Autodesk Inventor part; units mm, degrees
ref_plane "YZ Plane" through (0, 0, 0) normal (1, 0, 0) x (0, 1, 0)
ref_plane "XZ Plane" through (0, 0, 0) normal (0, 1, 0) x (-1, 0, 0)
ref_plane "XY Plane" through (0, 0, 0) normal (0, 0, 1) x (1, 0, 0)
sketch "スケッチ1" plane through (0, 0, 0) normal (0, 0, 1) x (1, 0, 0)
  line L0 (-22, 0) -> (22, 0)
  line L1 (22, 0) -> (22, 17)
  line L2 (22, 17) -> (-22, 17)
  line L3 (-22, 17) -> (-22, 0)
  point P0 (0, 0)
  point P1 (0, 0)
  dimension "d0" = 44
  dimension "d1" = 17
extrude "土台" add sketch "スケッチ1" along normal blind 2
sketch "スケッチ2" plane through (-22, 0, 0) normal (0, -1, 0) x (1, 0, 0)
  line L0 (22, 0) -> (22, 53.3234) construction
  circle A0 centre (22, 25) radius 15 construction
  line L1 (0, 2) -> (44, 2) construction
  line L2 (-7.4711, 25) -> (51.4711, 25) construction
  circle A1 centre (3.5, 25) radius 1.6
  circle A2 centre (40.5, 25) radius 1.6
  line L3 (0, 2) -> (7, 2)
  line L4 (7, 2) -> (7, 28.5)
  line L5 (7, 28.5) -> (0, 28.5)
  line L6 (0, 28.5) -> (0, 2)
  line L7 (44, 2) -> (37, 2)
  line L8 (37, 2) -> (37, 28.5)
  line L9 (37, 28.5) -> (44, 28.5)
  line L10 (44, 28.5) -> (44, 2)
  dimension "d4" = 30
  dimension "d5" = 23
  dimension "d6" = 3.2
  dimension "d7" = 37
  dimension "d8" = 3.5
extrude "モータ支柱" add sketch "スケッチ2" against normal blind 2
sketch "スケッチ3" plane through (22, 0, 0) normal (1, 0, 0) x (0, 0, -1)
  line L0 (-28.5, 0) -> (-28.5, 2)
  line L1 (-28.5, 0) -> (-28.5, 5)
  line L2 (-28.5, 5) -> (-2, 15)
  line L3 (-2, 17) -> (-2, 2)
  line L4 (0, 17) -> (0, 0)
  line L5 (0, 15) -> (-2, 15)
  line L6 (0, 0) -> (-28.5, 0)
  dimension "d11" = 5
  dimension "d12" = 15
extrude "補強リブ" add sketch "スケッチ3" along normal blind 2
mirror "ミラー1" about plane through (0, 0, 0) normal (1, 0, 0) of "補強リブ"
sketch "スケッチ4" plane through (0, 0, 2) normal (0, 0, 1) x (1, 0, 0)
  line L0 (0, 0) -> (0, 42.8792) construction
  line L1 (-15, 0) -> (15, 0) construction
  line L2 (22, 17) -> (-22, 17)
  point P0 (-17.5, 13)
  point P1 (17.5, 13)
  point P2 (0, 0)
  dimension "d15" = 35
  dimension "d24" = 4
hole "穴1" at (-17.5, 13, 2) at (17.5, 13, 2) direction (0, 0, -1) diameter 3.2 end through all
properties part number "SPG27_Braket"
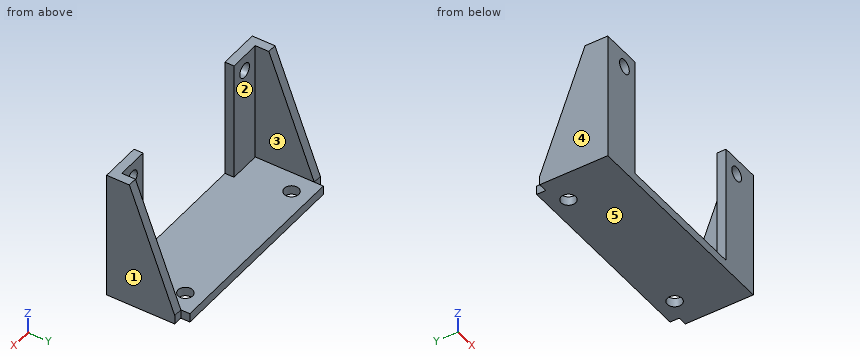
For this review, take the finished solid that the model builds, in its own axes (mm). Face numbers are marked on the shaded views. A direction names the side the tool comes from. Give positions to 0.01 mm unless a question says otherwise; leave off trailing zeros. Loops run counter-clockwise (first coordinate to the right, second up) from the corner with the lowest first, then second, coordinate; pieces in that order, holes last. Notation, with made-up numbers: M 65.25,34 L 108.25,34 A29 cw 108.25,73 Z; hole C -3,0 d4. An arc over 180 degrees is marked long. Put each result on its own line as item: value. Start each with the question number.
(1) For pin 1 (4 mm diameter, centred on x = -17.5, y = 13, fed in from -Z); pin 2 (5.5 mm diameter, centred on x = 18, z = 19, fed in from +Y); pin 3 (8.5 mm diameter, centred on x = -7.5, y = 6.5, fed in from +Z), all flat-tipped, find the tip position at first contact; note any pin that passes through.
(2) Add section D-D, the plane y = 3.5. Write out the cut boundary in (x, z).
(3) Machinability: for the marked faces 1 and 2, which of the approach directions +Z, -Z, +X, -X, +Y, -Y give a long, thin tool a straight path to every point of the face, cutting with its end or side? Answer none if there is none.
(4) The part is to be moulded in two halves that separate along X. For the marked faces 3, 4 and 5, say which applies: +X half, -X half, draft (parallel to the pull), parting line (faces both ways), or undercut.
(5) Add section B-B, the plane z = 25. Write out the cut boundary in (x, y), then the cut area to 3 significant figures.
(6) Add section A-A, the plane y = 13. Write out the cut boundary in (x, z).
(7) Wall thickness on L1, parallel to X at y = 2.75, z = 10.75; L2, parallel to Y at x = 17.5, z = 0.65; L3, parallel to Z at x = -18.5, y = 0.9: over which ranges is each line inside the solid? List them lowest first.
(8) Add section C-C, the plane z = 8.5. Write out the cut boundary in (x, y).
Result:
1. pin 1: stops at z = 0
1. pin 2: stops at y = 2
1. pin 3: stops at z = 2
2. outline: M -24,0 L 24,0 L 24,28.5 L 22,28.5 L 22,2 L -22,2 L -22,28.5 L -24,28.5 Z
3. face 1: +Z, -Z, +X, +Y, -Y
3. face 2: +Z, +Y
4. face 3: undercut
4. face 4: -X half
4. face 5: draft
5. outline: M -24,0 L -20.1,0 L -20.1,2 L -22,2 L -22,6.32 L -24,6.32 Z; M -16.9,0 L -15,0 L -15,2 L -16.9,2 Z; M 15,0 L 16.9,0 L 16.9,2 L 15,2 Z; M 20.1,0 L 24,0 L 24,6.32 L 22,6.32 L 22,2 L 20.1,2 Z
5. area: 40.5 mm^2
6. outline: M -24,0 L -19.1,0 L -19.1,2 L -22,2 L -22,7.3 L -24,7.3 Z; M -15.9,0 L 15.9,0 L 15.9,2 L -15.9,2 Z; M 19.1,0 L 24,0 L 24,7.3 L 22,7.3 L 22,2 L 19.1,2 Z
7. L1: x = -24 to -22, 22 to 24
7. L2: y = 0 to 11.4, 14.6 to 17
7. L3: z = 0 to 23.4, 26.6 to 28.5
8. outline: M -24,0 L -15,0 L -15,2 L -22,2 L -22,12.55 L -24,12.55 Z; M 15,0 L 24,0 L 24,12.55 L 22,12.55 L 22,2 L 15,2 Z
